Autodesk Inventor part; units mm, degrees
ref_plane "YZ Plane" through (0, 0, 0) normal (1, 0, 0) x (0, 1, 0)
ref_plane "XZ Plane" through (0, 0, 0) normal (0, 1, 0) x (-1, 0, 0)
ref_plane "XY Plane" through (0, 0, 0) normal (0, 0, 1) x (1, 0, 0)
sketch "Sketch1" plane through (0, 0, 0) normal (0, 0, 1) x (1, 0, 0)
  circle A0 centre (0, 0) radius 65
  dimension "d0" = 130
extrude "Extrusion1" add sketch "Sketch1" along normal blind 6
sketch "Sketch2" plane through (0, 0, 6) normal (0, 0, 1) x (1, 0, 0)
  circle A0 centre (0, 0) radius 65
  circle A1 centre (0, 0) radius 65
  circle A2 centre (0, 0) radius 59
  dimension "d3" = 6
extrude "Extrusion2" add sketch "Sketch2" along normal blind 50
sketch "Sketch3" plane through (0, 0, 56) normal (0, 0, 1) x (1, 0, 0)
  circle A0 centre (0, 0) radius 65
extrude "Extrusion3" add sketch "Sketch3" along normal blind 6
sketch "Sketch4" plane through (0, 0, 62) normal (0, 0, 1) x (1, 0, 0)
  line L0 (0, 0) -> (0, -36) construction
  line L1 (15, 14) -> (-15, 14)
  line L2 (-15, 14) -> (-15, -36)
  line L3 (-15, -36) -> (15, -36)
  line L4 (15, -36) -> (15, 14)
  point P0 (-15, 0)
  point P1 (0, 14)
  dimension "d25" = 36
  dimension "d26" = 50
  dimension "d27" = 30
extrude "Extrusion4" cut sketch "Sketch4" against normal blind 6
sketch "Sketch5" plane through (0, 0, 62) normal (0, 0, 1) x (1, 0, 0)
  line L0 (15, 25) -> (25, 25)
  line L1 (25, 25) -> (25, -5)
  line L2 (25, -5) -> (15, -5)
  line L3 (15, -5) -> (15, 25)
  point P0 (0, 0)
  dimension "d13" = 30
  dimension "d14" = 10
extrude "Extrusion5" [suppressed]
sketch "Sketch6" plane through (15, -25, 56) normal (-1, 0, 0) x (0, 0, 1)
  circle A0 centre (33, 23.5) radius 1
  circle A1 centre (33, 6.5) radius 1
  line L0 (36, 30) -> (36, 0)
  line L1 (33, 23.5) -> (33, 6.5) construction
  point P0 (-56, 25)
  point P1 (36, 15)
  point P2 (33, 15)
  dimension "d17" = 17
  dimension "d19" = 2
  dimension "d20" = 2
  dimension "d21" = 3
extrude "Extrusion6" [suppressed]
sketch "Sketch7" plane through (0, 0, 0) normal (0, 0, -1) x (-1, 0, 0)
  circle A0 centre (0, 0) radius 39.5
  dimension "d28" = 79
extrude "Extrusion7" cut sketch "Sketch7" against normal blind 5
sketch "Sketch8" plane through (0, 0, 5) normal (0, 0, -1) x (-1, 0, 0)
  circle A0 centre (-33, 0) radius 1.5
  point P0 (0, 0)
  dimension "d31" = 3
  dimension "d32" = 33
extrude "Extrusion8" cut sketch "Sketch8" against normal blind 5
pattern_circular "Circular Pattern1" count 12 over 360 about axis through (0, 0, 0) along (0, 0, 1) of "Extrusion8"
properties part number "per_base"
Verification items for the finished model (mm, model axes). A direction names the side the tool comes from. Give positions to 0.01 mm unless a question says otherwise; leave off trailing zeros. Order: outer loops, then holes, each group sorted by start corner. A loop starts at its lowest first (then second) coordinate and runs counter-clockwise, first axis right, second up. Notation, with made-up numbers: M -35.5,12.5 L -9.5,12.5 A22 cw -9.5,35.5 Z; hole C -31,-8 d3. An arc over 180 degrees is marked long. Answer as a JSON object with one key per item and string values. Group by question number.
1) Cross-section at C-C (z = 34). Enter the section's corners in (x, y), then the cut area to 3 significant figures.
2) Scan lines: line 1 along Z through (x, y) = (-18.5, -12); line 2 along Z through (x, y) = (-17.5, 38.5); line 3 along Y through (x, z) = (1, 42.5). Record each from-to range of solid material in increasing order. Write a range as [from, to].
3) Cross-section at D-D (y = 8). Enter the section's corners in (x, z).
4) Access from +Z, -Z, +X, -X, +Y, -Y to the whole of each face (thin tool, end or side, straight path). Record for faces 4 (the face through (16.175, -27.115, 5.493)), 5 (the face through (56.275, -17.722, 30.65)), 6 (the face through (0, 14, 59)).
5) Cross-section at B-B (y = 48.5). Enter the section's corners in (x, z), then the cut area to 3 significant figures.
6) Depth check by flat-ended pin: pin 1 Ø5 at (y, z) = (-22, 59.5) entering from -X; pin 2 Ø10 at (y, z) = (-6.5, 40) entering from -X; pin 3 Ø2.5 at (x, y) = (-28.58, 16.5) entering from -Z; pin 4 Ø2.5 at (x, y) = (0, -33) entering from -Z. Enter the tip coordinate at first touch or a pass-through.
7) Mould release check, pull along Z, two halves, no side actions. Record for faces 1 (the face through (29.11, 26.7, 2.46)), 2 (the face through (-1, 1, 6)), 3 (the face through (-1, -42, 0)): released by +Z, released by -Z, zero draft, split by the parting line, or undercut.
8) Cross-section at A-A (x = 49). Enter the section's corners in (y, z).
Result sheet:
{
 "1": {"outline": "C 0,0 d130; hole C 0,0 d118", "area": "2,340 mm2"},
 "2": {"line 1": "z = [5, 6], [56, 62]", "line 2": "z = [0, 6], [56, 62]", "line 3": "y = [-64.99, -58.99], [58.99, 64.99]"},
 "3": {"outline": "M -64.51,0 L -38.68,0 L -38.68,5 L 38.68,5 L 38.68,0 L 64.51,0 L 64.51,62 L 15,62 L 15,56 L 58.46,56 L 58.46,6 L -58.46,6 L -58.46,56 L -15,56 L -15,62 L -64.51,62 Z"},
 "4": {"face 4": "-Z", "face 5": "none", "face 6": "+Z"},
 "5": {"outline": "M -43.28,0 L 43.28,0 L 43.28,62 L -43.28,62 Z; hole M -33.6,6 L 33.6,6 L 33.6,56 L -33.6,56 Z", "area": "2,010 mm2"},
 "6": {"pin 1": "stops at x = -62.01", "pin 2": "stops at x = -64.98", "pin 3": "stops at z = 56", "pin 4": "passes through"},
 "7": {"face 1": "zero draft", "face 2": "undercut", "face 3": "released by -Z"},
 "8": {"outline": "M -42.71,0 L 42.71,0 L 42.71,62 L -42.71,62 Z; hole M -32.86,6 L 32.86,6 L 32.86,56 L -32.86,56 Z"}
}
